Verification items for the finished model (mm, model axes). Round coordinates to 2 decimals unless told otherwise and drop trailing zeros. Write each loop counter-clockwise with the first axis right and the second up, starting at its lowest first coordinate (ties: lowest second). Pieces come first, ordered by that corner, then holes. Notation, with made-up numbers: (22.25, 16) - (59.25, 16) arc R5 ccw to (59.25, 24) - close; hole circle Ø6 at (20.25, -26). An arc over 180 degrees is marked (long way). Answer as a JSON object with one key per item and string values. Group by question number.
1) Thickness scan on line 1 (Z direction, x = 35.5, y = -12.5); line 2 (X direction, y = -25.5, z = 38); line 3 (X direction, y = -3.5, z = 44.5). Record the ranges inside material, lowest first.
2) Section check A-A (z = 7). Enter the section's corners in (x, y).
3) Go/stop test with flat-tipped pins: pin 1 Ø1 at (y, z) = (-21.5, 39.5) entering from +X; pin 2 Ø8 at (x, y) = (0.5, -15.5) entering from +Z; pin 3 Ø2 at (x, z) = (-1, 46) entering from -Y. Record where each tip stops, or that it passes through.
```python
from build123d import *

# Parameters (mm, degrees)
F0_R     = 43.4220747745
F1_DEPTH = 25.4
F2_DEPTH = 32.512
F3_R     = 38.1


with BuildPart() as f1:
    # F0 (on Top) → F1 (new body)
    with BuildSketch(Plane.XY):
        Circle(F0_R)
    extrude(amount=F1_DEPTH)

    # F2 (add): a face of the model
    f2_faces = [f1.faces().sort_by_distance(p)[0] for p in [
        (0, 0, 25.4),
    ]]
    extrude(f2_faces, amount=F2_DEPTH)

    # F3
    f3_edges = [f1.edges().sort_by_distance(p)[0] for p in [
        (-43.422075, 0, 57.912),
    ]]
    fillet(f3_edges, radius=F3_R)


solid = f1.part
```
Returned:
{
 "1": {"line 1": "0 to 40", "line 2": "-29.24 to 29.24", "line 3": "-34.16 to 34.16"},
 "2": {"outline": "circle Ø86.84 at (0, 0)"},
 "3": {"pin 1": "x = 31.76", "pin 2": "z = 57.41", "pin 3": "y = -33.89"}
}
